Part model, mm, in its own coordinate system. A direction names the side the tool comes from. Give positions to 0.01 mm unless a question says otherwise; leave off trailing zeros. Order: outer loops, then holes, each group sorted by start corner. A loop starts at its lowest first (then second) coordinate and runs counter-clockwise, first axis right, second up. Notation, with made-up numbers: M 89.5,86 L 143.5,86 A14 ccw 143.5,102 Z; hole C 5,22 d11. An arc over 180 degrees is marked long. Write each question's results on one line, items separated by ' | '. Start each with the question number.
from build123d import *

# Parameters (mm, degrees)
SKETCH1_R           = 4
BOSS_EXTRUDE1_DEPTH = 10
SKETCH2_W           = 20
SKETCH2_H           = 20
SKETCH2_H_2         = 10
SKETCH2_W_2         = 40
BOSS_EXTRUDE2_DEPTH = 10
BOSS_EXTRUDE3_DEPTH = 35
SKETCH3_R           = 4
CUT_EXTRUDE1_DEPTH  = 59.309518948


with BuildPart() as part:
    # Sketch1 → Boss-Extrude1 (new body)
    with BuildSketch(Plane(origin=(0, 0, 0), x_dir=(1, 0, 0), z_dir=(0, 1, 0))):
        with BuildLine():
            Line((-30, -20), (30, -20))
            ThreePointArc((30, -20), (37.071067812, -17.071067812), (40, -10))
            Line((40, -10), (40, 20))
            Line((40, 20), (-40, 20))
            Line((-40, 20), (-40, -10))
            ThreePointArc((-40, -10), (-37.071067812, -17.071067812), (-30, -20))
        make_face()
        with Locations(Location((-30, -10, 0), (0, 0, 270))):
            Circle(SKETCH1_R, mode=Mode.SUBTRACT)
        with Locations(Location((30, -10, 0), (0, 0, 270))):
            Circle(SKETCH1_R, mode=Mode.SUBTRACT)
    extrude(amount=BOSS_EXTRUDE1_DEPTH)

    # Sketch2 → Boss-Extrude2 (add)
    with BuildSketch(Plane(origin=(0, 0, -20), x_dir=(-1, 0, 0), z_dir=(0, 0, -1))):
        with Locations((-30, 20)):
            Rectangle(SKETCH2_W, SKETCH2_H)
        with Locations((-30, 5)):
            Rectangle(SKETCH2_W, SKETCH2_H_2)
        with Locations((30, 20)):
            Rectangle(SKETCH2_W, SKETCH2_H)
        with Locations((30, 5)):
            Rectangle(SKETCH2_W, SKETCH2_H_2)
        with Locations((0, 5)):
            Rectangle(SKETCH2_W_2, SKETCH2_H_2)
    extrude(amount=-BOSS_EXTRUDE2_DEPTH)

    # Sketch2_3 → Boss-Extrude3 (add)
    with BuildSketch(Plane(origin=(0, 0, -20), x_dir=(-1, 0, 0), z_dir=(0, 0, -1))):
        with BuildLine():
            Line((-20, 10), (20, 10))
            Line((20, 10), (20, 30))
            Line((20, 30), (15, 30))
            ThreePointArc((15, 30), (0, 15), (-15, 30))
            Line((-15, 30), (-20, 30))
            Line((-20, 30), (-20, 10))
        make_face()
    extrude(amount=-BOSS_EXTRUDE3_DEPTH)

    # Sketch3 → Cut-Extrude1 (cut, through all)
    with BuildSketch(Plane.XY.offset(-10)):
        with Locations((30, 20)):
            Circle(SKETCH3_R)
        with Locations(Location((-30, 20, 0), (0, 0, 180))):
            Circle(SKETCH3_R)
    extrude(amount=-CUT_EXTRUDE1_DEPTH, mode=Mode.SUBTRACT)


solid = part.part
(1) Saw through at C-C on y = 8. Give the cut face in (x, z).
(2) Drop flat-ended pins along their axis: P1, Ø1.5, axis at x = -12.5, z = -15.5, coming from the +Y side; P2, Ø8, axis at x = 24.5, y = 26, coming from the +Z side; P3, Ø1, axis at y = 16.5, z = 2.5, coming from the -X side. Give the stop position or say it passes through.
(3) Saw through at D-D on x = 27. Give the cut face in (y, z).
(4) Probe L1, parallel to X at y = 2.5, z = 10; L2, parallel to Z at x = 25, y = 25.75; L3, parallel to Y at x = 26.5, z = -7. List the from-to ranges inside material, lowest first.
(5) Saw through at A-A on y = 17.25. Give the cut face in (x, z), plus the area to 3 significant figures.
(6) Saw through at B-B on z = -1.5. Give the cut face in (x, y), plus the area to 3 significant figures.
(7) Pull direction Z, two halves, no side cores. Call faces 6 (the cylindrical face through (36.99, 4.93, 17.15)), 7 (the cylindrical face through (33.966, 4.93, 9.479)), 8 (the cylindrical face through (-26.034, 4.93, 9.479)), 9 (the cylindrical face through (-27.05, 17.3, -14.93)): +Z half, -Z half, draft (parallel to the pull), parting line (faces both ways), or undercut.
(8) Tool access for faces 1 (the flat face through (-25, 20, -10)), 2 (the flat face through (0, 13, 15)), 3 (the flat face through (40, 12, -12)), 4 (the cylindrical face through (27.05, 22.7, -14.93)), 5 (the flat face through (20, 20, 2)): list every direction of +Z, -Z, +X, -X, +Y, -Y with a clear straight run to the whole face (end or side of a thin tool).
Taken from the geometry:
1) outline: M -40,-20 L 40,-20 L 40,10 A10 ccw 30,20 L -30,20 A10 ccw -40,10 Z; hole C -30,10 d8; hole C 30,10 d8
2) P1: stops at y = 22.97 | P2: stops at z = -10 | P3: stops at x = -20
3) outline: M 0,-20 L 17.35,-20 L 17.35,-10 L 10,-10 L 10,7.35 L 0,7.35 Z; M 0,12.65 L 10,12.65 L 10,20 L 0,20 Z; M 22.65,-20 L 30,-20 L 30,-10 L 22.65,-10 Z
4) L1: x = -40 to -34, -26 to 26, 34 to 40 | L2: z = -20 to -10 | L3: y = 0 to 10
5) outline: M -40,-20 L -32.9,-20 L -32.9,-10 L -40,-10 Z; M -27.1,-20 L -7.9,-20 L -7.9,15 L -20,15 L -20,-10 L -27.1,-10 Z; M 7.9,-20 L 27.1,-20 L 27.1,-10 L 20,-10 L 20,15 L 7.9,15 Z; M 32.9,-20 L 40,-20 L 40,-10 L 32.9,-10 Z | area: 1,130 mm²
6) outline: M -40,0 L 40,0 L 40,10 L 20,10 L 20,30 L 15,30 A15 cw -15,30 L -20,30 L -20,10 L -40,10 Z | area: 1,250 mm²
7) face 6: +Z half | face 7: undercut | face 8: undercut | face 9: draft
8) face 1: +Z, -X, +Y | face 2: +Z, +X, -X, +Y | face 3: +Z, -Z, +X, +Y, -Y | face 4: +Z, -Z | face 5: +Z, +X, +Y
